For this review, take the finished solid that the model builds, in its own axes (mm). Face numbers are marked on the shaded views. A direction names the side the tool comes from. Coordinates: 2 decimals unless noted, no trailing zeros. Loops run counter-clockwise (first coordinate to the right, second up) from the corner with the lowest first, then second, coordinate; pieces in that order, holes last. Notation, with made-up numbers: M -5,22.5 L 24,22.5 A33 cw 24,50.5 Z; hole C 36,46 d7. An arc over 180 degrees is marked long. Use one line per item in the form item = value.
```python
from build123d import *

# Parameters (mm, degrees)
CROQUIS1_R                   = 5
SALIENTE_EXTRUIR1_DEPTH      = 5
CROQUIS2_R                   = 1.7
SALIENTE_EXTRUIR2_DEPTH      = 5
TALADRO_DE_MARGEN_PARA_M61_D = 6.6


with BuildPart() as part:
    # Croquis1 → Saliente-Extruir1 (new body)
    with BuildSketch(Plane(origin=(0, 0, 0), x_dir=(1, 0, 0), z_dir=(0, 1, 0))):
        Circle(CROQUIS1_R)
    extrude(amount=SALIENTE_EXTRUIR1_DEPTH)

    # Croquis2 → Saliente-Extruir2 (add)
    with BuildSketch(Plane(origin=(0, 5, 0), x_dir=(1, 0, 0), z_dir=(0, 1, 0))):
        with BuildLine():
            ThreePointArc((-2.675283116, 9.6355), (-10, 0), (-2.675283116, -9.6355))
            ThreePointArc((-2.675283116, -9.6355), (0, -12.7), (2.675283116, -9.6355))
            ThreePointArc((2.675283116, -9.6355), (10, 0), (2.675283116, 9.6355))
            ThreePointArc((2.675283116, 9.6355), (0, 12.7), (-2.675283116, 9.6355))
        make_face()
        with Locations((0, 10)):
            Circle(CROQUIS2_R, mode=Mode.SUBTRACT)
        with Locations((0, -10)):
            Circle(CROQUIS2_R, mode=Mode.SUBTRACT)
    extrude(amount=SALIENTE_EXTRUIR2_DEPTH)

    # Taladro de margen para M61 (through all)
    with Locations(Plane(origin=(0, 0, 0), x_dir=(-1, 0, 0), z_dir=(0, -1, 0))):
        with Locations((0, 0)):
            Hole(TALADRO_DE_MARGEN_PARA_M61_D / 2)


solid = part.part
```
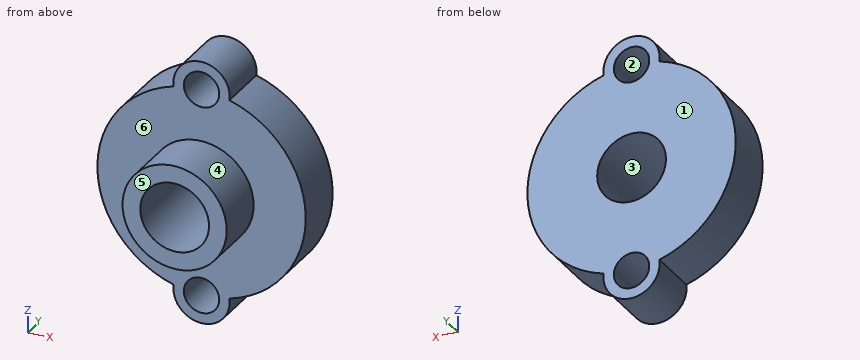
1. For pin 1 Ø1 at (y, z) = (7, 4.5) entering from -X; pin 2 Ø4 at (x, z) = (-4.5, -2.5) entering from -Y; pin 3 Ø5 at (x, y) = (-4, 5.5) entering from +Z (3 decimals); pin 4 Ø1 at (y, z) = (6.5, -3.5) entering from -X, all flat-tipped, find the tip position at first contact; note any pin that passes through.
Computed values:
pin_1 = -9.17
pin_2 = 0
pin_3 = 12.245
pin_4 = -9.54
2. Consider section D-D on z = 10. Write out the cut boundary in (x, y).
Computed values:
outline = M -2.7,5 L -1.7,5 L -1.7,10 L -2.7,10 Z; M 1.7,5 L 2.7,5 L 2.7,10 L 1.7,10 Z
3. Consider section B-B on y = 7. Write out the cut boundary in (x, z), plus the area to 3 significant figures.
Computed values:
outline = M -2.68,-9.64 A2.7 ccw long 2.68,-9.64 A10 ccw 2.68,9.64 A2.7 ccw long -2.68,9.64 A10 ccw Z; hole C 0,0 d6.6; hole C 0,-10 d3.4; hole C 0,10 d3.4
area = 286 mm2
4. Tool access review of the marked faces 5 and 6: name each direction out of +Z, -Z, +X, -X, +Y, -Y from which nothing blocks a thin tool from reaching the whole face with its end or side.
Computed values:
face_5 = +Z, -Z, +X, -X, -Y
face_6 = -Y
5. Consider section C-C on x = 0. Write out the cut boundary in (y, z), plus the area to 3 significant figures.
Computed values:
outline = M 0,-5 L 5,-5 L 5,-8.3 L 10,-8.3 L 10,-3.3 L 0,-3.3 Z; M 0,3.3 L 10,3.3 L 10,8.3 L 5,8.3 L 5,5 L 0,5 Z; M 5,-12.7 L 10,-12.7 L 10,-11.7 L 5,-11.7 Z; M 5,11.7 L 10,11.7 L 10,12.7 L 5,12.7 Z
area = 77.0 mm2
6. Wall thickness on line 1 along X through (y, z) = (7.4, 10); line 2 along Z through (x, y) = (0, 3.75); line 3 along Y through (x, z) = (3.5, 8.25): over which ranges is each line inside the solid? List them lowest first. Write a range as from..to.
Computed values:
line_1 = -2.7..-1.7, 1.7..2.7
line_2 = -5..-3.3, 3.3..5
line_3 = 5..10
7. Draft analysis for pull direction Z (two halves, no side actions). For the marked faces 1, 2, 3 and 4, state which applies: +Z half, -Z half, draft (parallel to the pull), parting line (faces both ways), or undercut.
Computed values:
face_1 = draft
face_2 = undercut
face_3 = undercut
face_4 = parting line
8. Consider section A-A on z = 0. Write out the cut boundary in (x, y).
Computed values:
outline = M -10,5 L -5,5 L -5,0 L -3.3,0 L -3.3,10 L -10,10 Z; M 3.3,0 L 5,0 L 5,5 L 10,5 L 10,10 L 3.3,10 Z
